Can you work these out from the drawing? Everything is in mm from the part's minimum corner. A direction names the side the tool comes from. Give positions to 0.01 mm unless a question says otherwise; leave off trailing zeros. Loops run counter-clockwise (first coordinate to the right, second up) from the corner with the lowest first, then second, coordinate; pieces in that order, holes last. Notation, with made-up numbers: (79.5, 82) - (136.5, 82) arc R31 cw to (136.5, 121) - close; hole circle Ø8 at (-15.5, 37.5). An arc over 180 degrees is marked (long way). One line per item, written item: value. Start each with the question number.
Q1. I want a section at A-A (z = 2.4). Please give me the cut outline in (x, y).
Q2. I want a section at C-C (y = 22.25). Please give me the cut outline in (x, z), then the cut area to 3 significant figures.
Q3. If I drill on line 1 (Y direction, x = 3.5, z = 4.3); line 2 (Z direction, x = 2.5, y = 26.5); line 3 (Z direction, x = 2.5, y = 20), over which ranges is the centre line in solid material (lowest first)? Write a range as from..to.
Q4. For the marked faces 1, 2 and 3, which set-ups out of +Z, -Z, +X, -X, +Y, -Y let a thin tool reach every point of the face, with its end or its side?
Q5. I'm going to push flat-ended pins straight in: P1, Ø1, axis at x = 1.5, y = 18.5, coming from the +Z side; P2, Ø1.5, axis at x = 4, y = 4, coming from the -Z side; P3, Ø2, axis at y = 5, z = 4, coming from the -X side. Where does each tip first touch, or does it pass through?
Q6. I want a section at B-B (x = 2.4). Please give me the cut outline in (y, z).
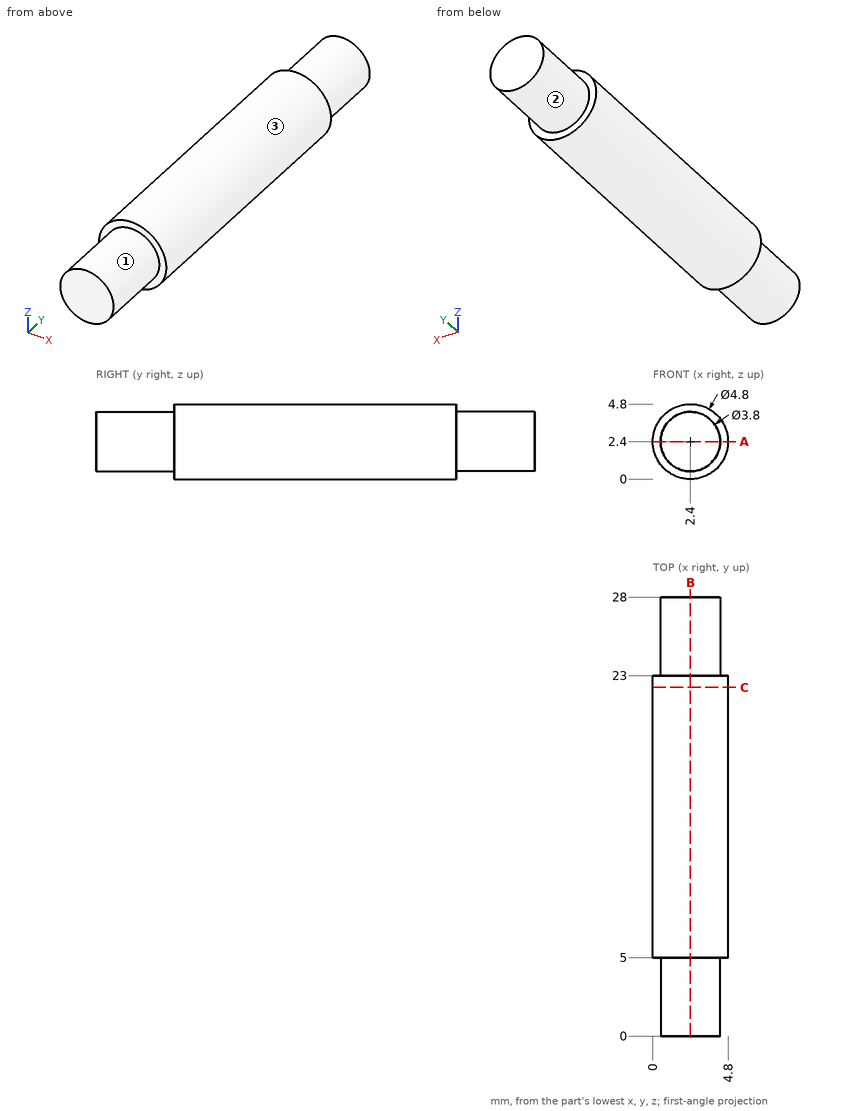
Worked answers:
1. outline: (0, 5) - (0.5, 5) - (0.5, 0) - (4.3, 0) - (4.3, 5) - (4.8, 5) - (4.8, 23) - (4.3, 23) - (4.3, 28) - (0.5, 28) - (0.5, 23) - (0, 23) - close
2. outline: circle Ø4.8 at (2.4, 2.4)
2. area: 18.1 mm²
3. line 1: y = 5..23
3. line 2: z = 0.5..4.3
3. line 3: z = 0..4.8
4. face 1: -Y
4. face 2: +Y
4. face 3: +Y, -Y
5. P1: stops at z = 4.77
5. P2: stops at z = 0.7
5. P3: stops at x = 0.08
6. outline: (0, 0.5) - (5, 0.5) - (5, 0) - (23, 0) - (23, 0.5) - (28, 0.5) - (28, 4.3) - (23, 4.3) - (23, 4.8) - (5, 4.8) - (5, 4.3) - (0, 4.3) - close
